Input: part model. Units: mm. Frame: model coordinates. A direction names the side the tool comes from. Round coordinates to 2 decimals unless told otherwise and drop trailing zeros. Order: outer loops, then holes, each group sorted by start corner. A loop starts at its lowest first (then second) coordinate and runs counter-clockwise, first axis right, second up.
Item 1: Reachability of faces 4 (the flat face through (-4, -67.405, 65)), 5 (the cylindrical face through (-1.217, -79.971, 62.942)), 6 (the cylindrical face through (-0.35, -13.06, 7.39)), 7 (the flat face through (0, -9, 15)) from +Z, -Z, +X, -X, +Y, -Y: full face, straight path, thin tool, end or side. Return the list, or none.
Item 2: Mould query, pull axis X, two halves, no side actions, for faces 1 (the cylindrical face through (-1.217, -68.638, 62.942)), 2 (the flat face through (-3, -66.805, 63)), 3 (the flat face through (-7.5, -53.3, 19.5)). Classes: released by +X, released by -X, zero draft, split by the parting line, or undercut.
Item 3: Cut plane A-A on y = -11.5. Output: boundary loops of the cut face in (x, z).
Item 4: Cut plane D-D on z = 73. Output: boundary loops of the cut face in (x, y).
Item 5: Line query: L1, parallel to X at y = 0, z = 6; L2, parallel to Y at x = 0, z = 6.5; L3, parallel to Y at x = 0, z = 10. Output: solid intervals per line, ascending.
Item 6: Cut plane B-B on x = 0. Give the number of separate pieces and of enclosed holes in the cut face, then the cut area to 3 significant figures.
Item 7: Cut plane C-C on y = 0. Output: boundary loops of the cut face in (x, z).
Item 8: First-contact query: pin 1 (7.5 mm diameter, centred on x = 1.5, y = -21, fed in from +Z); pin 2 (6.5 mm diameter, centred on x = 1, z = 65.5, fed in from +Y); pin 3 (4.5 mm diameter, centred on x = -1, z = 66, fed in from -Y); pin 4 (1 mm diameter, centred on y = 5, z = 16.5, fed in from -X). Flat tips, straight axial feed; report the tip coordinate or a pass-through.
```python
from build123d import *

# Parameters (mm, degrees)
BOSS_EXTRUDE1_DEPTH      = 7.5
BOSS_EXTRUDE1_DEPTH_BACK = 7.5
SKETCH3_R                = 2.25
CUT_EXTRUDE1_DEPTH       = 120.512655858
CUT_EXTRUDE2_DEPTH       = 106.882442604
CUT_EXTRUDE2_DEPTH_BACK  = 106.882442604
SKETCH4_R                = 2.1
SKETCH4_R_2              = 1.6


with BuildPart() as part:
    # Sketch1 → Boss-Extrude1 (new, two sides: drawn at the far end of the back side and taken through both)
    with BuildSketch(Plane(origin=(0, 0, 0), x_dir=(0, 0, -1), z_dir=(1, 0, 0)).offset(-BOSS_EXTRUDE1_DEPTH_BACK)):
        with BuildLine():
            Line((-15, 20), (0, 20))
            Line((0, 20), (0, -37.26819382))
            ThreePointArc((0, -37.26819382), (-13.04440593, -68.76017553), (-44.53638764, -81.80458146))
            Line((-44.53638764, -81.80458146), (-66.80458146, -81.80458146))
            Line((-66.80458146, -81.80458146), (-81.80458146, -81.80458146))
            Line((-81.80458146, -81.80458146), (-81.80458146, -66.80458146))
            Line((-81.80458146, -66.80458146), (-66.80458146, -66.80458146))
            Line((-66.80458146, -66.80458146), (-44.53638764, -66.80458146))
            ThreePointArc((-44.53638764, -66.80458146), (-23.651007648, -58.153573812), (-15, -37.26819382))
            Line((-15, -37.26819382), (-15, 20))
        make_face()
    extrude(amount=BOSS_EXTRUDE1_DEPTH + BOSS_EXTRUDE1_DEPTH_BACK)

    # Sketch3 → Cut-Extrude1 (cut, through all)
    with BuildSketch(Plane(origin=(0, -66.80458146, 0), x_dir=(1, 0, 0), z_dir=(0, 1, 0))):
        with Locations(Location((0, -66.80458146, 0), (0, 0, 270))):
            Circle(SKETCH3_R)
    extrude(amount=-CUT_EXTRUDE1_DEPTH, mode=Mode.SUBTRACT)

    # Sketch4 → Cut-Extrude2 (cut, two sides: drawn at the far end of the back side and taken through both)
    with BuildSketch(Plane.XY.offset(15).offset(-CUT_EXTRUDE2_DEPTH_BACK)):
        Circle(SKETCH4_R)
        with Locations((0, 11.5)):
            Circle(SKETCH4_R_2)
        with Locations((0, -11.5)):
            Circle(SKETCH4_R_2)
    extrude(amount=CUT_EXTRUDE2_DEPTH + CUT_EXTRUDE2_DEPTH_BACK, mode=Mode.SUBTRACT)

    # Sketch5 → Cut-Revolve1 (revolve, cut)
    with BuildSketch(Plane(origin=(0, 0, 0), x_dir=(0, 0, -1), z_dir=(1, 0, 0))):
        with BuildLine():
            Line((-62.75458146, -78.80458146), (-62.75458146, -81.10458146))
            ThreePointArc((-62.75458146, -81.10458146), (-62.725292138, -81.175292138), (-62.65458146, -81.20458146))
            Line((-62.65458146, -81.20458146), (-62.15458146, -81.20458146))
            Line((-62.15458146, -81.20458146), (-62.15458146, -81.80458146))
            Line((-62.15458146, -81.80458146), (-66.80458146, -81.80458146))
            Line((-66.80458146, -81.80458146), (-66.80458146, -78.80458146))
            Line((-66.80458146, -78.80458146), (-62.75458146, -78.80458146))
        make_face()
        with BuildLine():
            Line((-66.80458146, -69.80458146), (-62.75458146, -69.80458146))
            Line((-62.75458146, -69.80458146), (-62.75458146, -67.50458146))
            ThreePointArc((-62.75458146, -67.50458146), (-62.725292138, -67.433870782), (-62.65458146, -67.40458146))
            Line((-62.65458146, -67.40458146), (-62.15458146, -67.40458146))
            Line((-62.15458146, -67.40458146), (-62.15458146, -66.80458146))
            Line((-62.15458146, -66.80458146), (-66.80458146, -66.80458146))
            Line((-66.80458146, -66.80458146), (-66.80458146, -69.80458146))
        make_face()
    revolve(axis=Axis((0, -52.168735771, 66.80458146), (0, 1, 0)), mode=Mode.SUBTRACT)


solid = part.part
```
From the geometry:
1. face 4: +Y
1. face 5: -Y
1. face 6: +Z, -Z
1. face 7: +Z, +X, -X, +Y
2. face 1: undercut
2. face 2: zero draft
2. face 3: released by -X
3. outline: (-7.5, 0) - (-1.6, 0) - (-1.6, 15) - (-7.5, 15) - close; (1.6, 0) - (7.5, 0) - (7.5, 15) - (1.6, 15) - close
4. outline: (-7.5, -81.8) - (7.5, -81.8) - (7.5, -66.8) - (-7.5, -66.8) - close
5. L1: x = -7.5 to -2.1, 2.1 to 7.5
5. L2: y = -60.44 to -13.1, -9.9 to -2.1, 2.1 to 9.9, 13.1 to 20
5. L3: y = -65.39 to -13.1, -9.9 to -2.1, 2.1 to 9.9, 13.1 to 20
6. separate pieces: 5
6. enclosed holes: 0
6. area: 2,040 mm2
7. outline: (-7.5, 0) - (-2.1, 0) - (-2.1, 15) - (-7.5, 15) - close; (2.1, 0) - (7.5, 0) - (7.5, 15) - (2.1, 15) - close
8. pin 1: stops at z = 15
8. pin 2: stops at y = -66.8
8. pin 3: stops at y = -78.8
8. pin 4: passes through
